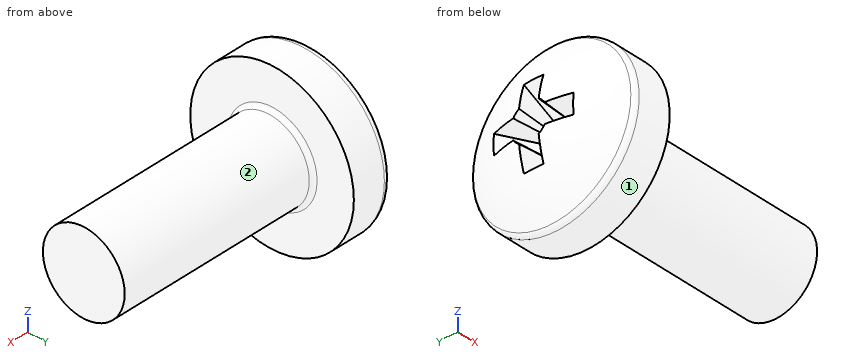
```python
from build123d import *

# Parameters (mm, degrees)
FILLET1_R    = 0.1
SKETCH3_W    = 0.48
SKETCH3_H    = 2.1
SKETCH4_W    = 0.48
SKETCH4_H    = 0.68402847
RECPAT_COUNT = 2
RECPAT_ANGLE = 90


with BuildPart() as part:
    # BodySke → Base-Revolve (revolve)
    with BuildSketch(Plane.XY):
        with BuildLine():
            Line((1.6, 1), (1.6, 2))
            Line((1.6, 2), (0.790020747, 2))
            ThreePointArc((0.790020747, 2), (0.709789294, 1.981130115), (0.646379599, 1.928476821))
            ThreePointArc((0.646379599, 1.928476821), (0.165895084, 1.016959861), (0, 0))
            Line((0, 0), (6.6, 0))
            Line((6.6, 0), (6.6, 1))
            Line((6.6, 1), (1.6, 1))
        make_face()
    revolve(axis=Axis((-25.4, 0, 0), (1, 0, 0)))

    # Fillet1
    fillet1_edges = [part.edges().sort_by_distance(p)[0] for p in [
        (1.6, -1, 0),
    ]]
    fillet(fillet1_edges, radius=FILLET1_R)

    # Sketch3 → Recess section 0
    with BuildSketch(Plane(origin=(0, 0, 0), x_dir=(0, 0, -1), z_dir=(1, 0, 0))):
        Rectangle(SKETCH3_W, SKETCH3_H)
    # Sketch4 → Recess section 1
    with BuildSketch(Plane(origin=(1.42, 0, 0), x_dir=(0, 0, -1), z_dir=(1, 0, 0))):
        Rectangle(SKETCH4_W, SKETCH4_H)
    recess = loft(mode=Mode.SUBTRACT)

    # RecPat: Recess ×2 about axis
    recpat_axis = Axis((0, 0, 0), (1, 0, 0))
    for i in range(1, RECPAT_COUNT):
        add(recess.rotate(recpat_axis, i * RECPAT_ANGLE / (RECPAT_COUNT - 1)), mode=Mode.SUBTRACT)

    # RecCorSke → RecessCore (revolve, cut)
    with BuildSketch(Plane.XY):
        Polygon((0, 0), (0, 0.454796073), (1.42, 0.3555), (1.535508952, 0), align=None)
    revolve(axis=Axis((-3.175, 0, 0), (1, 0, 0)), mode=Mode.SUBTRACT)


solid = part.part
```
Verification items for the finished model (mm, model axes). Face numbers are marked on the shaded views. A direction names the side the tool comes from. Coordinates: 2 decimals unless noted, no trailing zeros. Loops run counter-clockwise (first coordinate to the right, second up) from the corner with the lowest first, then second, coordinate; pieces in that order, holes last. Notation, with made-up numbers: (77.25, 44) -> (125.25, 44) arc R20 cw to (125.25, 57) -> close; hole circle Ø2 at (-9.5, 85.25). An arc over 180 degrees is marked (long way). Answer in a Markdown table with one row per item. Add a question column.
1. Access from +Z, -Z, +X, -X, +Y, -Y to the whole of each face (thin tool, end or side, straight path). Record for the marked faces 1 and 2.
2. Section check A-A, the plane x = 3.75. Enter the section's corners in (y, z), then the cut area to 3 significant figures.
3. Material ranges on probe 1 along Z at (x, y) = (4, 0.05); probe 2 along X at (y, z) = (-0.65, 0.45); probe 3 along Y at (x, z) = (0.5, -0.1), recorded low to high. Write a range as [from, to].
Derived:
| question | item | result |
|---|---|---|
| 1 | face 1 | +X, -X |
| 1 | face 2 | +X |
| 2 | outline | circle Ø2 at (0, 0) |
| 2 | area | 3.14 mm² |
| 3 | probe 1 | z = [-1, 1] |
| 3 | probe 2 | x = [0.1, 6.6] |
| 3 | probe 3 | y = [-1.71, -0.8], [0.8, 1.71] |
